Check sheet for the drawn part. Datum: minimum x, y, z corner. Units: mm. Round coordinates to 2 decimals unless told otherwise and drop trailing zeros. Write each loop counter-clockwise with the first axis right and the second up, starting at its lowest first coordinate (ties: lowest second). Pieces come first, ordered by that corner, then holes.
Item 1: Cross-section at C-C on y = 1.6. Enter the section's corners in (x, z).
Item 2: Cross-section at A-A on z = 45. Enter the section's corners in (x, y).
Item 3: Go/stop test with flat-tipped pins: pin 1 Ø2 at (y, z) = (2, 53) entering from -X; pin 2 Ø4.5 at (x, z) = (10.3, 40) entering from -Y; pin 3 Ø1.5 at (x, y) = (29, 1.5) entering from +Z; pin 4 Ø2 at (x, y) = (60.5, 1) entering from -Z. Record where each tip stops, or that it passes through.
Item 4: Cross-section at D-D on x = 22. Enter the section's corners in (y, z).
Item 5: Material ranges on line 1 (Z direction, x = 45, y = 0.9); line 2 (X direction, y = 1.8, z = 40); line 3 (Z direction, x = 59, y = 1.4), recorded low to high.
Item 6: Cross-section at B-B on x = 10.3. Enter the section's corners in (y, z).
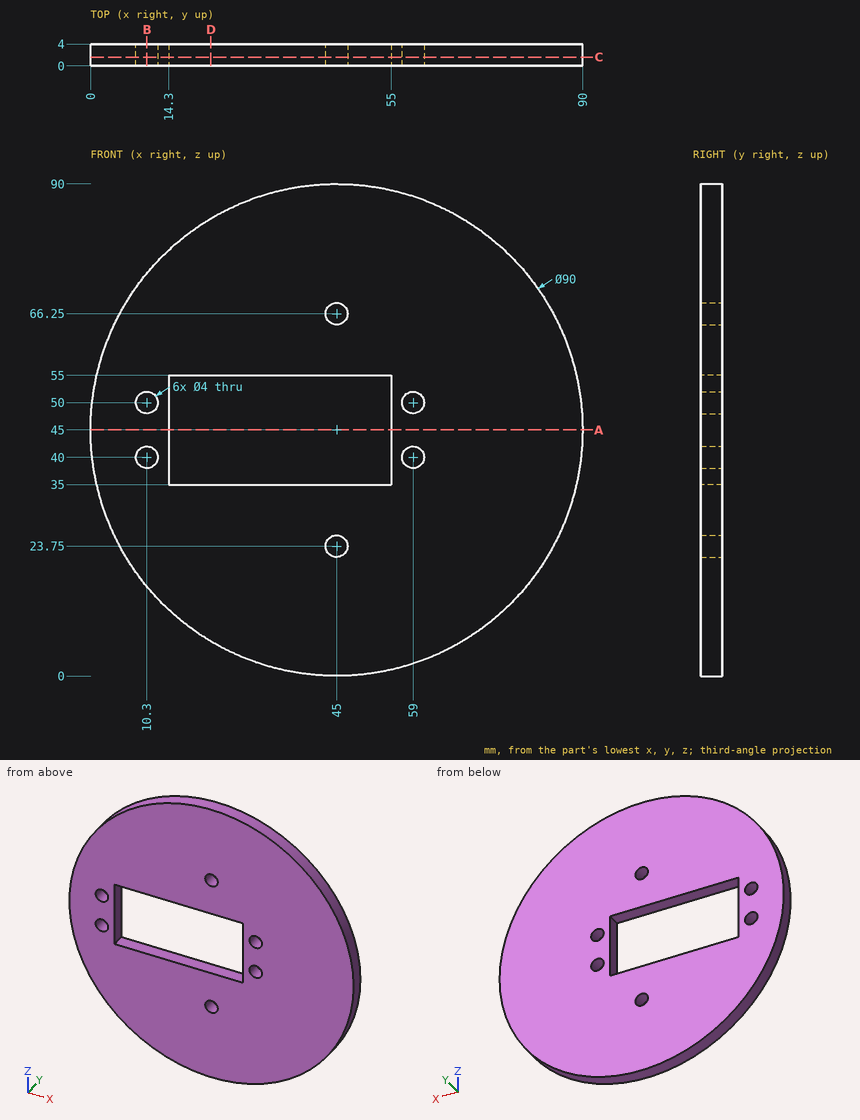
Response values:
1. outline: circle Ø90 at (45, 45); hole circle Ø4 at (10.3, 40); hole circle Ø4 at (10.3, 50); hole (14.3, 35) - (55, 35) - (55, 55) - (14.3, 55) - close; hole circle Ø4 at (45, 23.75); hole circle Ø4 at (45, 66.25); hole circle Ø4 at (59, 40); hole circle Ø4 at (59, 50)
2. outline: (0, 0) - (14.3, 0) - (14.3, 4) - (0, 4) - close; (55, 0) - (90, 0) - (90, 4) - (55, 4) - close
3. pin 1: stops at x = 0.55
3. pin 2: stops at y = 0
3. pin 3: stops at z = 87.34
3. pin 4: stops at z = 2.4
4. outline: (0, 6.32) - (4, 6.32) - (4, 35) - (0, 35) - close; (0, 55) - (4, 55) - (4, 83.68) - (0, 83.68) - close
5. line 1: z = 0 to 21.75, 25.75 to 35, 55 to 64.25, 68.25 to 90
5. line 2: x = 0.28 to 8.3, 12.3 to 14.3, 55 to 57, 61 to 89.72
5. line 3: z = 2.23 to 38, 42 to 48, 52 to 87.77
6. outline: (0, 16.35) - (4, 16.35) - (4, 38) - (0, 38) - close; (0, 42) - (4, 42) - (4, 48) - (0, 48) - close; (0, 52) - (4, 52) - (4, 73.65) - (0, 73.65) - close
